For this review, take the finished solid that the model builds, in its own axes (mm). A direction names the side the tool comes from. Round coordinates to 2 decimals unless told otherwise and drop trailing zeros. Order: outer loops, then holes, each group sorted by start corner. A loop starts at its lowest first (then second) coordinate and runs counter-clockwise, first axis right, second up. Notation, with made-up numbers: M 59,49 L 92,49 A12 cw 92,56 Z; hole C 17.5,83 d11. An arc over 180 degrees is marked long. Answer as a JSON object with one key per item and string values.
from build123d import *

# Parameters (mm, degrees)
F0_W          = 400.05
F0_H          = 285.75
F0_W_2        = 336.55
F0_H_2        = 222.25
F1_DEPTH      = 5.55625
F3_DEPTH      = 142.876
F3_DEPTH_BACK = 142.876
F5_DEPTH      = 200.026
F5_DEPTH_BACK = 200.026


with BuildPart() as f1:
    # F0 (on Front) → F1 (new body, symmetric)
    with BuildSketch(Plane.XZ):
        Rectangle(F0_W, F0_H)
        Rectangle(F0_W_2, F0_H_2, mode=Mode.SUBTRACT)
    extrude(amount=F1_DEPTH, both=True)

    # F2 (on Top) → F3 (cut, two sides)
    with BuildSketch(Plane.XY) as f3_sk:
        with BuildLine():
            ThreePointArc((-187.325, -5.55625), (-191.0729853256, -4.6678735007), (-194.1626797348, -2.3677875757))
            ThreePointArc((-194.1626797348, -2.3677875757), (-197.5840837344, -0.5984369952), (-200.025, 2.38125))
            Line((-200.025, 2.38125), (-200.025, -5.55625))
            Line((-200.025, -5.55625), (-187.325, -5.55625))
        make_face()
        with BuildLine():
            Line((194.1626797348, -2.3677875757), (187.325, -5.55625))
            ThreePointArc((187.325, -5.55625), (191.0729853256, -4.6678735007), (194.1626797348, -2.3677875757))
        make_face()
        with BuildLine():
            ThreePointArc((194.1626797348, -2.3677875757), (191.0729853256, -4.6678735007), (187.325, -5.55625))
            Line((187.325, -5.55625), (200.025, -5.55625))
            Line((200.025, -5.55625), (200.025, 2.38125))
            ThreePointArc((200.025, 2.38125), (197.5840837344, -0.5984369952), (194.1626797348, -2.3677875757))
        make_face()
        with BuildLine():
            Line((200.025, 2.38125), (194.1626797348, -2.3677875757))
            ThreePointArc((194.1626797348, -2.3677875757), (197.5840837344, -0.5984369952), (200.025, 2.38125))
        make_face()
    extrude(amount=-F3_DEPTH, mode=Mode.SUBTRACT)
    extrude(f3_sk.sketch, amount=F3_DEPTH_BACK, mode=Mode.SUBTRACT)

    # F4 (on Right) → F5 (cut, two sides)
    with BuildSketch(Plane.YZ) as f5_sk:
        with BuildLine():
            Line((-5.55625, 142.875), (-5.55625, 130.175))
            ThreePointArc((-5.55625, 130.175), (-4.6678735007, 133.9229853256), (-2.3677875757, 137.0126797348))
            ThreePointArc((-2.3677875757, 137.0126797348), (-0.5984369952, 140.4340837344), (2.38125, 142.875))
            Line((2.38125, 142.875), (-5.55625, 142.875))
        make_face()
        with BuildLine():
            ThreePointArc((-2.3677875757, -137.0126797348), (-4.6678735007, -133.9229853256), (-5.55625, -130.175))
            Line((-5.55625, -130.175), (-5.55625, -142.875))
            Line((-5.55625, -142.875), (2.38125, -142.875))
            ThreePointArc((2.38125, -142.875), (-0.5984369952, -140.4340837344), (-2.3677875757, -137.0126797348))
        make_face()
        with BuildLine():
            Line((-2.3677875757, -137.0126797348), (-5.55625, -130.175))
            ThreePointArc((-5.55625, -130.175), (-4.6678735007, -133.9229853256), (-2.3677875757, -137.0126797348))
        make_face()
        with BuildLine():
            Line((2.38125, -142.875), (-2.3677875757, -137.0126797348))
            ThreePointArc((-2.3677875757, -137.0126797348), (-0.5984369952, -140.4340837344), (2.38125, -142.875))
        make_face()
    extrude(amount=-F5_DEPTH, mode=Mode.SUBTRACT)
    extrude(f5_sk.sketch, amount=F5_DEPTH_BACK, mode=Mode.SUBTRACT)


solid = f1.part
1) Add section B-B on z = 75. State the section outline as (x, y) points (3 decimals), and give its area (3 significant figures).
Geometry check:
{"outline": "M -200.025,2.381 A9.525 ccw -194.163,-2.368 A9.525 ccw -187.325,-5.556 L -168.275,-5.556 L -168.275,5.556 L -200.025,5.556 Z; M 168.275,-5.556 L 187.325,-5.556 L 194.163,-2.368 L 200.025,2.381 L 200.025,5.556 L 168.275,5.556 Z", "area": "627 mm²"}
2) For L1, parallel to Z at x = 61, y = 4.75 (3 decimals); L2, parallel to X at y = 4.75, z = -79.5 (3 decimals); L3, parallel to X at y = -3.75, z = -53 (3 decimals), list the stretches that pass through material, from the lowest coordinate up.
Geometry check:
{"L1": "z = -142.875 to -111.125, 111.125 to 142.875", "L2": "x = -200.025 to -168.275, 168.275 to 200.025", "L3": "x = -192.634 to -168.275, 168.275 to 191.199"}
3) Machinability: for faces 3 (the flat face through (-168.275, 0, -2)), 4 (the flat face through (-3, 5.556, -125)), which of the approach directions +Z, -Z, +X, -X, +Y, -Y give a long, thin tool a straight path to every point of the face, cutting with its end or side? Answer none if there is none.
Geometry check:
{"face 3": "+Y, -Y", "face 4": "+Z, -Z, +X, -X, +Y"}
4) Add section A-A on x = -160. State the section outline as (y, z) points (3 decimals), and give its area (3 significant figures).
Geometry check:
{"outline": "M -5.556,-130.175 L -2.368,-137.013 L 2.381,-142.875 L 5.556,-142.875 L 5.556,-111.125 L -5.556,-111.125 Z; M -5.556,111.125 L 5.556,111.125 L 5.556,142.875 L 2.381,142.875 A9.525 ccw -2.368,137.013 A9.525 ccw -5.556,130.175 Z", "area": "627 mm²"}
5) Add section C-C on y = -0.25. State the section outline as (x, z) points (3 decimals).
Geometry check:
{"outline": "M -197.99,-139.627 L 196.777,-139.627 L 196.777,140.84 L -197.99,140.84 Z; hole M -168.275,-111.125 L 168.275,-111.125 L 168.275,111.125 L -168.275,111.125 Z"}
6) Insertion check: P1, Ø4, axis at x = -157.5, y = -4, coming from the +Z side; P2, Ø3.5, axis at x = -42.5, y = 0, coming from the +Z side; P3, Ø1, axis at y = -1, z = 58, coming from the -X side. Each pin has a flat end and moves straight along its axis. Give the tip position at first contact, or say it passes through.
Geometry check:
{"P1": "stops at z = 138.08", "P2": "stops at z = 142.51", "P3": "stops at x = -197.7"}
7) Mouldability with a two-part tool opening along X and no side actions: class faces 1 (the flat face through (-15, -5.556, -115)), 2 (the flat face through (-2, 0, -111.125)) as +X half, -X half, draft (parallel to the pull), parting line (faces both ways), or undercut.
Geometry check:
{"face 1": "draft", "face 2": "undercut"}
